Read the model definition and answer for the solid it produces. Units are mm, in the model's axes. A direction names the side the tool comes from. Coordinates: 2 decimals unless noted, no trailing zeros. Write each loop counter-clockwise with the first axis right and the second up, starting at its lowest first coordinate (ties: lowest second). Pieces come first, ordered by that corner, then holes. Notation, with made-up numbers: (56, 74) -> (108, 74) arc R18 ccw to (108, 86) -> close; hole circle Ø4 at (19.25, 17). An arc over 180 degrees is marked (long way). Answer as a JSON object with one key per item and string values. Group by question number.
(1) Which of the six approach directions +Z, -Z, +X, -X, +Y, -Y give full straight-line access (tool end or side, diameter ignored) to faces 4 (the face through (150, -3.9, 0)), 5 (the face through (150, 0, 3.9)), 6 (the face through (150, 0, -3.9))?
(2) For a pull along Z with two mould halves and no side action, classify faces 1 (the face through (150, -6, -10)), 2 (the face through (150, -10, 6)), 3 (the face through (150, 3.9, 0)) as +Z half, -Z half, draft (parallel to the pull), parting line (faces both ways), or undercut.
(3) Straight lines are drawn through the part: L1, parallel to Z at x = 211, y = 0; L2, parallel to Z at x = 240.5, y = -7.75; L3, parallel to Y at x = 127.5, z = 8.75. For each, find the intervals that lie inside material, in ascending order.
(4) Flat-ended cylindrical pins translate along their axes: P1, Ø12, axis at y = -4.5, z = -3, coming from the +X side; P2, Ø3, axis at x = 147.5, z = -0.5, coming from the -Y side; P3, Ø0.5, axis at x = 152, y = -9, coming from the +Z side; P4, Ø1, axis at x = 215, y = 3, coming from the +Z side. Find the tip coordinate at first contact, or state that the pin passes through.
(5) Find section A-A (y = 0). Give the vertices of the cut face in (x, z).
from build123d import *

# Parameters (mm, degrees)
SKETCH1_R                = 2.5
F_20_X_20_X_R1_5_1_DEPTH = 305


with BuildPart() as part:
    # Sketch1 → 铝型材 20 X 20 X R1.5(1) (new body)
    with BuildSketch(Plane.YZ):
        with BuildLine():
            Line((-3.6, 10), (-3.6, 9.5))
            Line((-3.6, 9.5), (-3.1, 9.5))
            Line((-3.1, 9.5), (-3.1, 8.5))
            Line((-3.1, 8.5), (-5.5, 8.5))
            Line((-5.5, 8.5), (-5.5, 6.65))
            Line((-5.5, 6.65), (-2.75, 3.9))
            Line((-2.75, 3.9), (2.75, 3.9))
            Line((2.75, 3.9), (5.5, 6.65))
            Line((5.5, 6.65), (5.5, 8.5))
            Line((5.5, 8.5), (3.1, 8.5))
            Line((3.1, 8.5), (3.1, 9.5))
            Line((3.1, 9.5), (3.6, 9.5))
            Line((3.6, 9.5), (3.6, 10))
            Line((3.6, 10), (8.5, 10))
            ThreePointArc((8.5, 10), (9.560660172, 9.560660172), (10, 8.5))
            Line((10, 8.5), (10, 3.6))
            Line((10, 3.6), (9.5, 3.6))
            Line((9.5, 3.6), (9.5, 3.1))
            Line((9.5, 3.1), (8.5, 3.1))
            Line((8.5, 3.1), (8.5, 5.5))
            Line((8.5, 5.5), (6.65, 5.5))
            Line((6.65, 5.5), (3.9, 2.75))
            Line((3.9, 2.75), (3.9, -2.75))
            Line((3.9, -2.75), (6.65, -5.5))
            Line((6.65, -5.5), (8.5, -5.5))
            Line((8.5, -5.5), (8.5, -3.1))
            Line((8.5, -3.1), (9.5, -3.1))
            Line((9.5, -3.1), (9.5, -3.6))
            Line((9.5, -3.6), (10, -3.6))
            Line((10, -3.6), (10, -8.5))
            ThreePointArc((10, -8.5), (9.560660172, -9.560660172), (8.5, -10))
            Line((8.5, -10), (3.6, -10))
            Line((3.6, -10), (3.6, -9.5))
            Line((3.6, -9.5), (3.1, -9.5))
            Line((3.1, -9.5), (3.1, -8.5))
            Line((3.1, -8.5), (5.5, -8.5))
            Line((5.5, -8.5), (5.5, -6.65))
            Line((5.5, -6.65), (2.75, -3.9))
            Line((2.75, -3.9), (-2.75, -3.9))
            Line((-2.75, -3.9), (-5.5, -6.65))
            Line((-5.5, -6.65), (-5.5, -8.5))
            Line((-5.5, -8.5), (-3.1, -8.5))
            Line((-3.1, -8.5), (-3.1, -9.5))
            Line((-3.1, -9.5), (-3.6, -9.5))
            Line((-3.6, -9.5), (-3.6, -10))
            Line((-3.6, -10), (-8.5, -10))
            ThreePointArc((-8.5, -10), (-9.560660172, -9.560660172), (-10, -8.5))
            Line((-10, -8.5), (-10, -3.6))
            Line((-10, -3.6), (-9.5, -3.6))
            Line((-9.5, -3.6), (-9.5, -3.1))
            Line((-9.5, -3.1), (-8.5, -3.1))
            Line((-8.5, -3.1), (-8.5, -5.5))
            Line((-8.5, -5.5), (-6.65, -5.5))
            Line((-6.65, -5.5), (-3.9, -2.75))
            Line((-3.9, -2.75), (-3.9, 2.75))
            Line((-3.9, 2.75), (-6.65, 5.5))
            Line((-6.65, 5.5), (-8.5, 5.5))
            Line((-8.5, 5.5), (-8.5, 3.1))
            Line((-8.5, 3.1), (-9.5, 3.1))
            Line((-9.5, 3.1), (-9.5, 3.6))
            Line((-9.5, 3.6), (-10, 3.6))
            Line((-10, 3.6), (-10, 8.5))
            ThreePointArc((-10, 8.5), (-9.560660172, 9.560660172), (-8.5, 10))
            Line((-8.5, 10), (-3.6, 10))
        make_face()
        Circle(SKETCH1_R, mode=Mode.SUBTRACT)
    extrude(amount=F_20_X_20_X_R1_5_1_DEPTH)


solid = part.part
Results below:
{
 "1": {"face 4": "+X, -X, -Y", "face 5": "+Z, +X, -X", "face 6": "-Z, +X, -X"},
 "2": {"face 1": "-Z half", "face 2": "draft", "face 3": "undercut"},
 "3": {"L1": "z = -3.9 to -2.5, 2.5 to 3.9", "L2": "z = -10 to -5.5, 5.5 to 10", "L3": "y = -9.98 to -3.1, 3.1 to 9.98"},
 "4": {"P1": "stops at x = 305", "P2": "stops at y = -3.9", "P3": "stops at z = 9.98", "P4": "stops at z = 9.5"},
 "5": {"outline": "(0, -3.9) -> (305, -3.9) -> (305, -2.5) -> (0, -2.5) -> close; (0, 2.5) -> (305, 2.5) -> (305, 3.9) -> (0, 3.9) -> close"}
}
